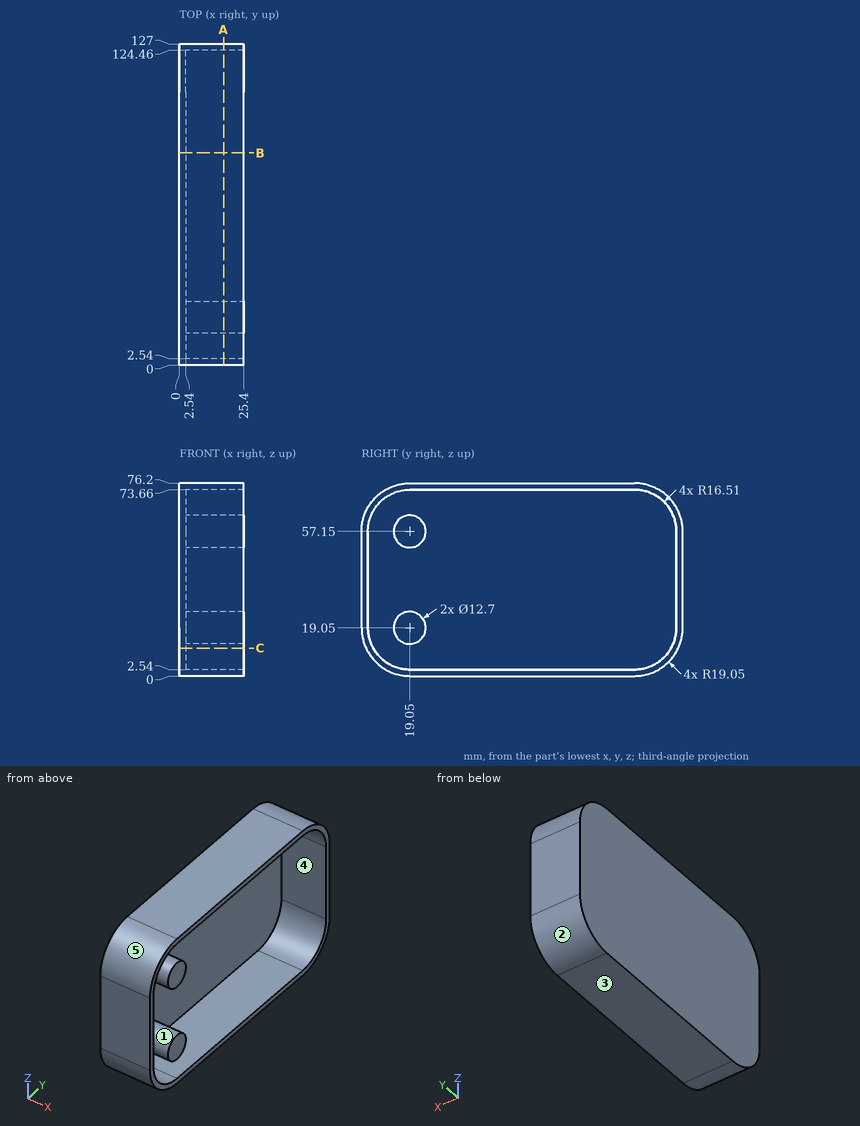
Geometry: see drawing. Coordinates: mm, zero at the bounding-box minimum. A direction names the side the tool comes from. Give positions to 0.01 mm unless a question says otherwise; leave off trailing zeros. Order: outer loops, then holes, each group sorted by start corner. A loop starts at its lowest first (then second) coordinate and runs counter-clockwise, first axis right, second up. Notation, with made-up numbers: (86, 72.25) - (105, 72.25) arc R16 ccw to (105, 90.25) - close; hole circle Ø3 at (79, -13.75). An arc over 180 degrees is marked (long way). One line per item, written item: value.
1. Line query: probe 1 along Z at (x, y) = (8.25, 66); probe 2 along Y at (x, z) = (6, 19); probe 3 along Y at (x, z) = (16.5, 40). Output: solid intervals per line, ascending.
Determined:
probe 1: 0 to 2.54, 73.66 to 76.2
probe 2: 0 to 2.54, 12.7 to 25.4, 124.46 to 127
probe 3: 0 to 2.54, 124.46 to 127
2. Draft query along Z for the marked faces 3, 4 and 5. Return one class per face: released by +Z, released by -Z, zero draft, split by the parting line, or undercut.
Determined:
face 3: released by -Z
face 4: undercut
face 5: released by +Z
3. Cut plane A-A, the plane x = 17.5. Output: boundary loops of the cut face in (y, z), and give its area (3 significant figures).
Determined:
outline: (0, 19.05) arc R19.05 ccw to (19.05, 0) - (107.95, 0) arc R19.05 ccw to (127, 19.05) - (127, 57.15) arc R19.05 ccw to (107.95, 76.2) - (19.05, 76.2) arc R19.05 ccw to (0, 57.15) - close; circle Ø12.7 at (19.05, 19.05); circle Ø12.7 at (19.05, 57.15); hole (2.54, 19.05) arc R16.51 ccw to (19.05, 2.54) - (107.95, 2.54) arc R16.51 ccw to (124.46, 19.05) - (124.46, 57.15) arc R16.51 ccw to (107.95, 73.66) - (19.05, 73.66) arc R16.51 ccw to (2.54, 57.15) - close
area: 1,180 mm2
4. Cut plane C-C, the plane z = 11. Output: boundary loops of the cut face in (x, y), and give its area (3 significant figures).
Determined:
outline: (0, 1.78) - (25.4, 1.78) - (25.4, 4.64) - (2.54, 4.64) - (2.54, 122.36) - (25.4, 122.36) - (25.4, 125.22) - (0, 125.22) - close
area: 444 mm2
5. Reachability of the marked faces 1 and 2 from +Z, -Z, +X, -X, +Y, -Y: full face, straight path, thin tool, end or side. Return the list, or none.
Determined:
face 1: +X
face 2: -Z, +X, -X, +Y
6. Pin query (flat end, axial travel): pin 1 Ø7 at (x, y) = (17.5, 73.5) entering from -Z; pin 2 Ø1.5 at (x, z) = (12, 67.5) entering from +Y; pin 3 Ø1.5 at (y, z) = (96.5, 18.5) entering from +X. Return the tip coordinate at first contact, or that it passes through.
Determined:
pin 1: z = 0
pin 2: y = 124.4
pin 3: x = 2.54
7. Cut plane B-B, the plane y = 84. Output: boundary loops of the cut face in (x, z).
Determined:
outline: (0, 0) - (25.4, 0) - (25.4, 2.54) - (2.54, 2.54) - (2.54, 73.66) - (25.4, 73.66) - (25.4, 76.2) - (0, 76.2) - close
